Source: CAD feature listing. Evaluate the final solid. Frame: model axes, mm. Face numbers are marked on the shaded views. A direction names the side the tool comes from. Give positions to 0.01 mm unless a question says otherwise; leave off trailing zeros. Loops run counter-clockwise (first coordinate to the right, second up) from the corner with the lowest first, then second, coordinate; pieces in that order, holes last.
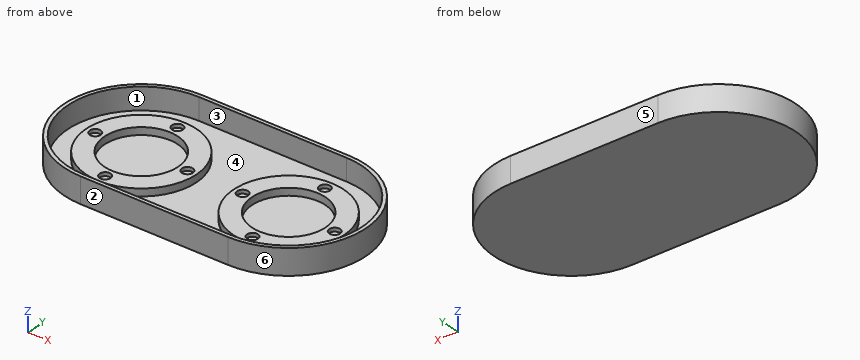
Solid Edge part; units mm, degrees
sketch "Sketch1" plane through (0, 0, 0) normal (0, 0, 1) x (1, 0, 0)
  line L0 (20, -21) -> (-20, -21)
  line L1 (-20, 21) -> (20, 21)
  arc A0 (20, 21) -> (20, -21) centre (20, 0) cw
  arc A1 (-20, -21) -> (-20, 21) centre (-20, 0) cw
extrude "Protrusion1" add sketch "Sketch1" against normal blind 7
sketch "Sketch2" plane through (0, 0, 0) normal (0, 0, 1) x (1, 0, 0)
  arc A0 (-20, -20) -> (-20, 20) centre (-20, 0) cw
  line L0 (-20, -20) -> (20, -20)
  arc A1 (20, 20) -> (20, -20) centre (20, 0) cw
  line L1 (-20, 20) -> (20, 20)
extrude "VaciadoExtruido_1" cut sketch "Sketch2" against normal blind 6
sketch "Sketch3" plane through (0, 0, -6) normal (0, 0, 1) x (1, 0, 0)
  circle A0 centre (-20, 0) radius 10
  circle A1 centre (-20, 0) radius 15
  circle A2 centre (20, 0) radius 15
  circle A3 centre (20, 0) radius 10
extrude "Protrusion2" add sketch "Sketch3" along normal blind 2
sketch "Sketch4" plane through (-20, 0, -4) normal (0, 0, 1) x (1, 0, 0)
  circle A0 centre (0, 12.5) radius 1.5
  circle A1 centre (-12.5, 0) radius 1.5
  circle A2 centre (0, -12.5) radius 1.5
  circle A3 centre (12.5, 0) radius 1.5
extrude "VaciadoExtruido_2" cut sketch "Sketch4" against normal blind 1
mirror "Mirror1" about plane through (0, 0, 0) normal (1, 0, 0) of "VaciadoExtruido_2"
(1) Section A-A, the plane z = -1.5. Return the cut outline in (x, y).
A:
outline: (-20, -21) - (20, -21) arc R21 ccw to (20, 21) - (-20, 21) arc R21 ccw to start; hole (-20, -20) - (20, -20) arc R20 ccw to (20, 20) - (-20, 20) arc R20 ccw to start
(2) First-contact query: pin 1 (0.9 mm diameter, centred on x = 33, y = -0.5, fed in from +Z); pin 2 (1 mm diameter, centred on y = 8, z = -2.5, fed in from +X); pin 3 (8 mm diameter, centred on x = -5, y = -1, fed in from +Z). Flat tips, straight axial feed; report the tip coordinate or a pass-through.
A:
pin 1: stops at z = -5
pin 2: stops at x = 39.62
pin 3: stops at z = -4
(3) Reachability of the marked faces 1 and 2 from +Z, -Z, +X, -X, +Y, -Y: full face, straight path, thin tool, end or side. Return the list, or none.
A:
face 1: +Z
face 2: +Z, -Z, +X, -X, -Y
(4) Mould query, pull axis Y, two halves, no side actions, for the marked faces 3, 4, 5 and 6. Classes: pulls with the +Y half, pulls with the -Y half, needs draft (parallel to the pull), parting line crosses it, or undercut.
A:
face 3: undercut
face 4: undercut
face 5: pulls with the +Y half
face 6: parting line crosses it
(5) Ray query, line 1 along Y through (x, z) = (-20, -4.75); line 2 along Y through (x, z) = (13, -3.5); line 3 along Y through (x, z) = (-32.5, -4.4). Return the intervals inside material, ascending.
A:
line 1: y = -21 to -20, -15 to -14, -11 to -10, 10 to 11, 14 to 15, 20 to 21
line 2: y = -21 to -20, 20 to 21
line 3: y = -16.87 to -15.61, -8.29 to -1.5, 1.5 to 8.29, 15.61 to 16.87
(6) Section B-B, the plane x = -7.5. Return the cut outline in (y, z), then the cut area to 3 significant figures.
A:
outline: (-21, -7) - (21, -7) - (21, 0) - (20, 0) - (20, -6) - (8.29, -6) - (8.29, -4) - (1.5, -4) - (1.5, -5) - (-1.5, -5) - (-1.5, -4) - (-8.29, -4) - (-8.29, -6) - (-20, -6) - (-20, 0) - (-21, 0) - close
area: 84.2 mm2
(7) Section D-D, the plane x = 15.5. Return the cut outline in (y, z), then the cut area to 3 significant figures.
A:
outline: (-21, -7) - (21, -7) - (21, 0) - (20, 0) - (20, -6) - (14.31, -6) - (14.31, -4) - (8.93, -4) - (8.93, -6) - (-8.93, -6) - (-8.93, -4) - (-14.31, -4) - (-14.31, -6) - (-20, -6) - (-20, 0) - (-21, 0) - close
area: 75.5 mm2
(8) Section C-C, the plane y = 12.5. Return the cut outline in (x, z), then the cut area to 3 significant figures.
A:
outline: (-36.87, -7) - (36.87, -7) - (36.87, 0) - (35.61, 0) - (35.61, -6) - (28.29, -6) - (28.29, -4) - (21.5, -4) - (21.5, -5) - (18.5, -5) - (18.5, -4) - (11.71, -4) - (11.71, -6) - (-11.71, -6) - (-11.71, -4) - (-18.5, -4) - (-18.5, -5) - (-21.5, -5) - (-21.5, -4) - (-28.29, -4) - (-28.29, -6) - (-35.61, -6) - (-35.61, 0) - (-36.87, 0) - close
area: 149 mm2
